The model under review builds one solid part; all positions refer to its coordinate system, in mm. Round coordinates to 2 decimals unless told otherwise and drop trailing zeros. Order: outer loops, then holes, each group sorted by start corner. A loop starts at its lowest first (then second) coordinate and runs counter-clockwise, first axis right, second up. Notation, with made-up numbers: M -16,-6 L 36,-6 A35 cw 36,27 Z; hole C 18.25,29.5 d9. An arc over 180 degrees is marked long. Answer as CSV lines item,"result". Start each with the question number.
Autodesk Inventor part; units mm, degrees
ref_plane "YZ Plane" through (0, 0, 0) normal (1, 0, 0) x (0, 1, 0)
ref_plane "XZ Plane" through (0, 0, 0) normal (0, 1, 0) x (-1, 0, 0)
ref_plane "XY Plane" through (0, 0, 0) normal (0, 0, 1) x (1, 0, 0)
sketch "Sketch1" plane through (0, 0, 0) normal (0, 1, 0) x (-1, 0, 0)
  line L0 (-1.8331, -3.175) -> (-3.6662, 0)
  line L1 (-3.6662, 0) -> (-1.8331, 3.175)
  line L2 (-1.8331, 3.175) -> (1.8331, 3.175)
  line L3 (1.8331, 3.175) -> (3.6662, 0)
  line L4 (3.6662, 0) -> (1.8331, -3.175)
  line L5 (1.8331, -3.175) -> (-1.8331, -3.175)
  point P0 (0, 0)
  point P1 (0, 0)
  dimension "d0" = 6.35
extrude "Body" add sketch "Sketch1" along normal blind 6.35
sketch "Sketch2" plane through (0, 6.35, 0) normal (0, 1, 0) x (1, 0, 0)
  circle A0 centre (0, 0) radius 2.0955
  dimension "d3" = 4.191
extrude "Hole 2" [suppressed]
sketch "Sketch3" plane through (0, 0, 0) normal (0, -1, 0) x (1, 0, 0)
  circle A0 centre (0, 0) radius 2.0955
  dimension "d6" = 4.191
extrude "Hole 1" cut sketch "Sketch3" against normal blind 12.7
chamfer "Hole 2 Chamfer 1" [suppressed]
chamfer "Hole 1 Chamfer 1" distance 0.127 distance2 0.1244 1 edges at (-2.0955, 0, 0) measured on face at (-0.0842, 0, 2.8101)
sketch "Sketch4" plane through (0, 0, 0) normal (0, 0, 1) x (1, 0, 0)
  line L0 (1.8331, 6.35) -> (-1.8331, 6.35)
  line L1 (0, 6.35) -> (-3.0353, 6.35)
  line L2 (-3.6662, 6.35) -> (-1.8331, 6.35)
  line L3 (-3.6662, 0) -> (-3.6662, 6.35)
  arc A0 (-3.0353, 6.35) -> (-3.6662, 5.715) centre (-2.2234, 4.9124) ccw
  line L4 (-3.6662, 5.715) -> (-6.3588, 8.3147)
  line L5 (-6.3588, 8.3147) -> (0, 6.35)
  line L6 (0, 6.35) -> (0, -3.486)
  point P0 (0, 0)
  dimension "d15" = 3.0353
  dimension "d16" = 1.651
  dimension "d17" = 0.635
revolve "Hole 2 Chamfer 2" [suppressed]
sketch "Sketch5" plane through (0, 0, 0) normal (0, 0, 1) x (1, 0, 0)
  line L0 (0, 0) -> (-3.0353, 0)
  line L1 (1.8331, 0) -> (-1.8331, 0)
  line L2 (-3.6662, 0) -> (-3.6662, 6.35)
  arc A0 (-3.6662, 0.635) -> (-3.0353, 0) centre (-2.2234, 1.4376) ccw
  line L3 (0, 0) -> (0, -2.1986)
  line L4 (-3.6662, 0.635) -> (-4.1154, -0.8715)
  line L5 (-4.1154, -0.8715) -> (0, 0)
  point P0 (-3.6662, 18.415)
  dimension "d19" = 3.0353
  dimension "d20" = 1.651
  dimension "d21" = 0.635
revolve "Hole 1 Chamfer 2" cut sketch "Sketch5" angle 360 about axis through (0, 0, 0) along (0, -1, 0)
chamfer "Hole 2 Chamfer 1 For Short" distance 0.127 distance2 0.1244 1 edges at (-2.0955, 6.35, 0) measured on face at (-0.0842, 6.35, 2.8101)
sketch "Sketch7" plane through (0, 0, 0) normal (0, 0, 1) x (1, 0, 0)
  line L0 (0, 6.3504) -> (3.0353, 6.35)
  line L1 (3.6662, 6.35) -> (1.8331, 6.35)
  line L2 (3.6662, 0.635) -> (3.6662, 6.35)
  arc A0 (3.6662, 5.715) -> (3.0353, 6.35) centre (2.2234, 4.9124) ccw
  line L3 (3.6662, 5.715) -> (4.2663, 7.2532)
  line L4 (4.2663, 7.2532) -> (0, 6.3504)
  line L5 (0, 8.1561) -> (0, 6.3504)
  line L6 (1.8331, 6.35) -> (-1.8331, 6.35)
  point P0 (0, 0)
  point P1 (0, 6.35)
  dimension "d33" = 3.0353
  dimension "d34" = 1.651
  dimension "d35" = 0.635
revolve "Hole 2 Chamfer 2 For Short" cut sketch "Sketch7" angle 360 about axis through (0, 8.1561, 0) along (0, -1, 0)
properties part number "Standoff .5" material "VEX Aluminum Alloy 5052-H32"
Item 1: Consider section B-B (y = 2.5). State the section outline as (x, z) points (1 decimal), and give its area (3 significant figures).
Item 2: The part is to be moulded in two halves that separate along Z. For faces 1 (the cylindrical face through (2, 3.13, 0.63)), 2 (the flat face through (2.737, 3.132, -1.61)), 3 (the flat face through (2, 6.35, 2)), 4 (the flat face through (2.76, 3.13, 1.57)), say which applies: +Z half, -Z half, draft (parallel to the pull), parting line (faces both ways), or undercut.
Item 3: Wall thickness on probe 1 along Z at (x, y) = (0, 3.25) (1 decimal); probe 2 along Z at (x, y) = (0.75, 2.5) (3 decimals); probe 3 along X at (y, z) = (5.75, 1.75): over which ranges is each line inside the solid? List them lowest first. Write a range as [from, to].
Reported:
1,outline,"M -3.7,0 L -1.8,-3.2 L 1.8,-3.2 L 3.7,0 L 1.8,3.2 L -1.8,3.2 Z; hole C 0,0 d4.2"
1,area,"21.1 mm²"
2,face 1,"undercut"
2,face 2,"-Z half"
2,face 3,"draft"
2,face 4,"+Z half"
3,probe 1,"z = [-3.2, -2.1], [2.1, 3.2]"
3,probe 2,"z = [-3.175, -1.957], [1.957, 3.175]"
3,probe 3,"x = [-2.66, -1.15], [1.15, 2.66]"
